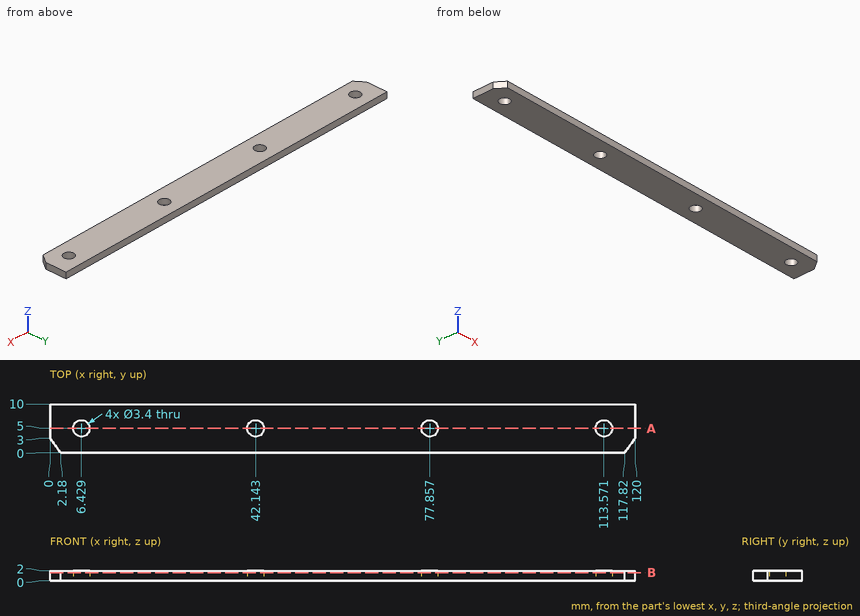
Here's the drawing with two shaded views (mm, measured from the low corner). I have some questions. Coordinates: 2 decimals unless noted, no trailing zeros. Order: outer loops, then holes, each group sorted by start corner. A loop starts at its lowest first (then second) coordinate and runs counter-clockwise, first axis right, second up.
Item 1: If we section it at A-A, the plane y = 5: List the corners of the cut face in (x, z) for me, then the cut area to 3 significant figures.
Response values:
outline: (0, 0) - (4.73, 0) - (4.73, 2) - (0, 2) - close; (8.13, 0) - (40.44, 0) - (40.44, 2) - (8.13, 2) - close; (43.84, 0) - (76.16, 0) - (76.16, 2) - (43.84, 2) - close; (79.56, 0) - (111.87, 0) - (111.87, 2) - (79.56, 2) - close; (115.27, 0) - (120, 0) - (120, 2) - (115.27, 2) - close
area: 213 mm2
Item 2: If we section it at B-B, the plane z = 1.6: List the corners of the cut face in (x, y) for me.
Response values:
outline: (0, 3) - (2.18, 0) - (117.82, 0) - (120, 3) - (120, 10) - (0, 10) - close; hole circle Ø3.4 at (6.43, 5); hole circle Ø3.4 at (42.14, 5); hole circle Ø3.4 at (77.86, 5); hole circle Ø3.4 at (113.57, 5)
Item 3: I'm going to push flat-ended pins straight in: pin 1 Ø1 at (x, z) = (31.5, 0.5) entering from -Y; pin 2 Ø3 at (x, y) = (113.57, 5) entering from +Z (3 decimals). Where does each tip first touch, or does it pass through?
Response values:
pin 1: stops at y = 0
pin 2: passes through
Item 4: I need wall thicknesses on probe 1 along X at (y, z) = (6.5, 1.1) (1 decimal); probe 2 along X at (y, z) = (5.5, 1.15) (1 decimal); probe 3 along Y at (x, z) = (79, 0.35). Which ranges of each line are inside material? Lowest first, please.
Response values:
probe 1: x = 0 to 5.6, 7.2 to 41.3, 42.9 to 77.1, 78.7 to 112.8, 114.4 to 120
probe 2: x = 0 to 4.8, 8.1 to 40.5, 43.8 to 76.2, 79.5 to 111.9, 115.2 to 120
probe 3: y = 0 to 3.74, 6.26 to 10
